Read the model definition and answer for the solid it produces. Units are mm, in the model's axes. Round coordinates to 2 decimals unless told otherwise and drop trailing zeros. Write each loop counter-clockwise with the first axis right and the second up, starting at its lowest first coordinate (ties: lowest second). Pieces come first, ordered by that corner, then holes. Notation, with made-up numbers: (-13, 69) -> (3, 69) arc R11 cw to (3, 86) -> close; hole circle Ø4 at (33, -14.5). An arc over 180 degrees is marked (long way). Return JSON: item names as keys, results as strings. Group by question number.
(1) Straight lines are drawn through the part: line 1 (X direction, y = 43, z = 4.05); line 2 (X direction, y = 44, z = 3); line 3 (X direction, y = 16.5, z = 4.1). For each, find the intervals that lie inside material, in ascending order.
(2) A cutting plane is placed at B-B on y = 17.5. Give the vertices of the cut face in (x, z).
(3) A cutting plane is placed at A-A on z = 2.7. Give the vertices of the cut face in (x, y).
(4) Given pin 1 (1.9 mm diameter, centred on x = 60.05, y = 43.31, fed in from +Z), flat-ended and moving along its own axis, determine where the tip first touches the part or whether it passes through.
(5) The mould has two halves that part along X. Classify faces 1 (the cylindrical face through (30.87, 42.23, 2.46)), 2 (the cylindrical face through (61.574, 42.83, 2.465)), 3 (the flat face through (24.048, 29, 2)), 4 (the flat face through (46, 47.31, 2)): released by +X, released by -X, zero draft, split by the parting line, or undercut.
Autodesk Fusion 360 part; units mm, degrees
sketch "Schizzo1" plane through (0, 0, 0) normal (0, 0, 1) x (1, 0, 0)
  line L0 (24.0483, 47.3102) -> (68.0483, 47.3102)
  line L1 (68.0483, 47.3102) -> (68.0483, 12.1102)
  line L2 (68.0483, 12.1102) -> (24.0483, 12.1102)
  line L3 (24.0483, 12.1102) -> (24.0483, 47.3102)
  line L4 (46.0483, 47.3102) -> (46.0483, 12.1102) construction
  line L5 (24.0483, 43.3102) -> (68.0483, 43.3102) construction
  circle A0 centre (46.0483, 15.3102) radius 1.4
  circle A1 centre (32.0483, 43.3102) radius 1.6
  circle A2 centre (60.0483, 43.3102) radius 1.6
  line L6 (59.5483, 12.1102) -> (68.0483, 20.7102)
  dimension "d1" = 44
  dimension "d2" = 35.2
  dimension "d3" = 2.8
  dimension "d4" = 4
  dimension "d6" = 28
  dimension "d7" = 3.2
  dimension "d8" = 28
  dimension "d9" = 8.5
  dimension "d10" = 8.6
extrude "Estrusione1" add sketch "Schizzo1" along normal blind 5 contours L0 L1 L2 L3 L6
Checks:
{
 "1": {"line 1": "x = 24.05 to 30.48, 33.62 to 58.48, 61.62 to 68.05", "line 2": "x = 24.05 to 30.6, 33.49 to 58.6, 61.49 to 68.05", "line 3": "x = 24.05 to 45.31, 46.79 to 63.89"},
 "2": {"outline": "(24.05, 0) -> (64.88, 0) -> (64.88, 5) -> (24.05, 5) -> close"},
 "3": {"outline": "(24.05, 12.11) -> (59.55, 12.11) -> (68.05, 20.71) -> (68.05, 47.31) -> (24.05, 47.31) -> close; hole circle Ø3.2 at (32.05, 43.31); hole circle Ø2.8 at (46.05, 15.31); hole circle Ø3.2 at (60.05, 43.31)"},
 "4": {"pin 1": "passes through"},
 "5": {"face 1": "undercut", "face 2": "undercut", "face 3": "released by -X", "face 4": "zero draft"}
}
